Part print with two shaded views. Sizes in mm from the minimum x, y, z corner. A direction names the side the tool comes from. Give positions to 0.01 mm unless a question says otherwise; leave off trailing zeros. Write each loop counter-clockwise with the first axis right and the second up, starting at its lowest first coordinate (ties: lowest second). Pieces come first, ordered by that corner, then holes.
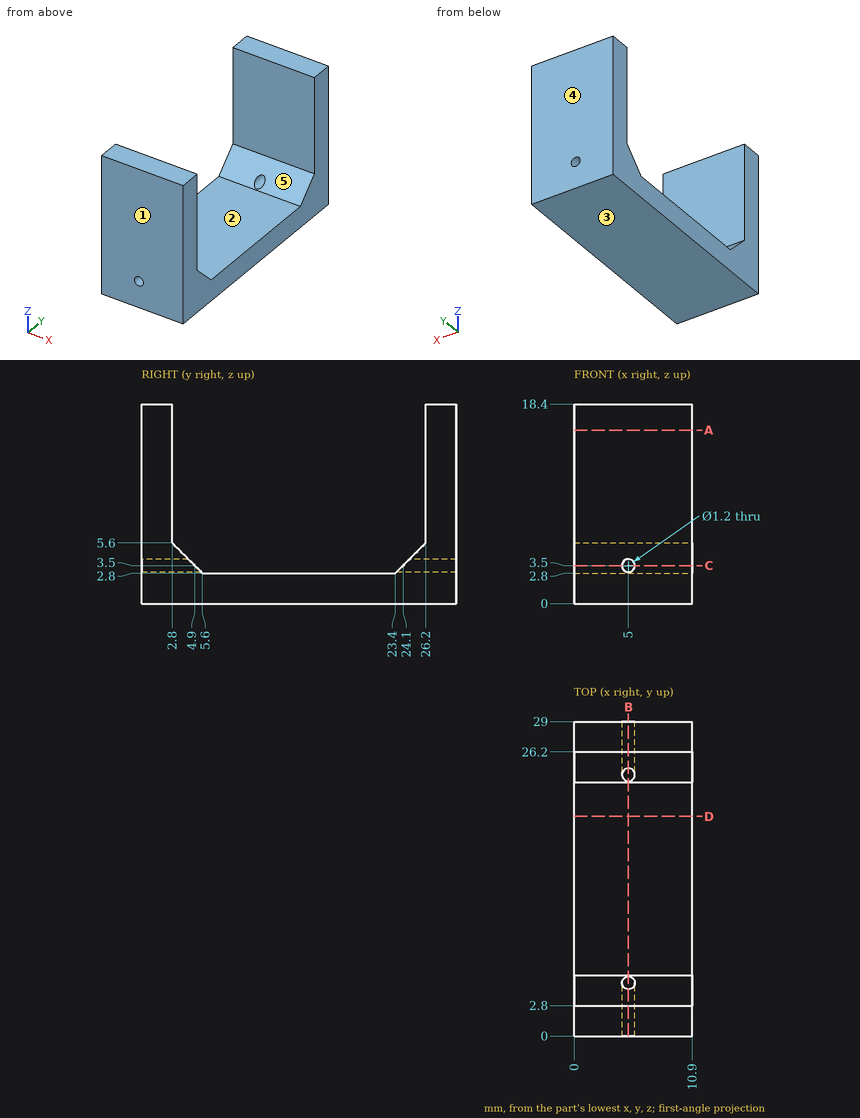
1) Flat gauge pin, fed straight in: P1, Ø5.5, axis at x = 3, y = 18, coming from the +Z side. Where does the tip first touch, or does it go through?
Check result:
P1: stops at z = 2.8
2) Saw through at C-C (z = 3.5). Write the cut outline in (x, y).
Check result:
outline: (0, 0) - (4.4, 0) - (4.4, 4.9) - (0, 4.9) - close; (0, 24.1) - (4.4, 24.1) - (4.4, 29) - (0, 29) - close; (5.6, 0) - (10.9, 0) - (10.9, 4.9) - (5.6, 4.9) - close; (5.6, 24.1) - (10.9, 24.1) - (10.9, 29) - (5.6, 29) - close
3) Saw through at A-A (z = 16). Write the cut outline in (x, y), and give its area (3 significant figures).
Check result:
outline: (0, 0) - (10.9, 0) - (10.9, 2.8) - (0, 2.8) - close; (0, 26.2) - (10.9, 26.2) - (10.9, 29) - (0, 29) - close
area: 61.0 mm2
4) Saw through at D-D (y = 20.25). Write the cut outline in (x, z), and give its area (3 significant figures).
Check result:
outline: (0, 0) - (10.9, 0) - (10.9, 2.8) - (0, 2.8) - close
area: 30.5 mm2
5) Drill centre lines: L1, parallel to X at y = 3.55, z = 3.5; L2, parallel to Y at x = 8.5, z = 9.5; L3, parallel to Z at x = 5, y = 2.75. Where is each one in solid material? Low to high.
Check result:
L1: x = 0 to 4.4, 5.6 to 10.9
L2: y = 0 to 2.8, 26.2 to 29
L3: z = 0 to 2.9, 4.1 to 18.4
6) 3-axis set-ups, long thin cutter, end or side, ignore diameter. For the marked faces 4 and 5: which of +Z, -Z, +X, -X, +Y, -Y reach the whole face in a straight line?
Check result:
face 4: +Z, -Z, +X, -X, +Y
face 5: +Z, +X, -X
7) Mould opens along Y. For the marked faces 1, 2 and 3 say: +Y half, -Y half, draft (parallel to the pull), parting line (faces both ways), or undercut.
Check result:
face 1: -Y half
face 2: undercut
face 3: draft
8) Saw through at B-B (x = 5). Write the cut outline in (y, z).
Check result:
outline: (0, 0) - (29, 0) - (29, 2.9) - (23.5, 2.9) - (23.4, 2.8) - (5.6, 2.8) - (5.5, 2.9) - (0, 2.9) - close; (0, 4.1) - (4.3, 4.1) - (2.8, 5.6) - (2.8, 18.4) - (0, 18.4) - close; (24.7, 4.1) - (29, 4.1) - (29, 18.4) - (26.2, 18.4) - (26.2, 5.6) - close
